```python
from build123d import *

# Parameters (mm, degrees)
CYLINDER009_R            = 2.2
CYLINDER009_DEPTH        = 20
ARRAY006_Z_COUNT         = 3
ARRAY006_Z_PITCH         = 10
CYLINDER008_R            = 1.8
CYLINDER008_DEPTH        = 10
ARRAY005_X_COUNT         = 2
ARRAY005_X_PITCH         = 20
ARRAY005_Y_COUNT         = 2
ARRAY005_Y_PITCH         = 20
ARRAY005_PLACEMENT_ANGLE = 90
PAD002_DEPTH             = 16


with BuildPart() as holder_insert_hole_array:
    # Cylinder009 → Cylinder009 (new body)
    with BuildSketch(Plane.XZ):
        Circle(CYLINDER009_R)
    extrude(amount=CYLINDER009_DEPTH)

    # Array006 Z: holder insert hole array ×3


with BuildPart() as holder_insert_hole_array_1:
    add(holder_insert_hole_array.part)
    with Locations(*[(0, 0, i * ARRAY006_Z_PITCH) for i in range(1, ARRAY006_Z_COUNT)]):
        add(holder_insert_hole_array.part)


with BuildPart() as holder_insert_hole_array_2:
    # Array006 placement: moved
    add(holder_insert_hole_array_1.part.moved(Location((35, 103, 71.5))))


with BuildPart() as holder_hole_fusion:
    # Cylinder008 → Cylinder008 (new body)
    with BuildSketch(Plane.XY):
        Circle(CYLINDER008_R)
    extrude(amount=CYLINDER008_DEPTH)

    # Array005 X: holder hole fusion ×2


with BuildPart() as holder_hole_fusion_1:
    add(holder_hole_fusion.part)
    with Locations(*[(i * ARRAY005_X_PITCH, 0, 0) for i in range(1, ARRAY005_X_COUNT)]):
        add(holder_hole_fusion.part)

    # Array005 Y: holder hole fusion ×2


with BuildPart() as holder_hole_fusion_2:
    add(holder_hole_fusion_1.part)
    with Locations(*[(0, i * ARRAY005_Y_PITCH, 0) for i in range(1, ARRAY005_Y_COUNT)]):
        add(holder_hole_fusion_1.part)


with BuildPart() as holder_hole_fusion_3:
    # Array005 placement: moved
    add(holder_hole_fusion_2.part.moved(Location((24, 88, 16))).rotate(Axis((24, 88, 16), (1, 0, 0)), ARRAY005_PLACEMENT_ANGLE))

    # Fusion008: union holder insert hole array
    add(holder_insert_hole_array_2.part)


with BuildPart() as holder_cut:
    # Sketch002 → Pad002 (new body, symmetric)
    with BuildSketch(Plane.YZ):
        with BuildLine():
            Line((65.267053, 48), (83, 48))
            Line((83, 48), (83, 9.6))
            Line((83, 9.6), (87, 9.6))
            Line((87, 9.6), (87, 40.719632))
            ThreePointArc((94.280368, 48), (89.13237, 45.86763), (87, 40.719632))
            Line((94.280368, 48), (95.267053, 48))
            Line((95.267053, 48), (95.267053, 98))
            ThreePointArc((95.267053, 98), (92.767053, 100.5), (90.267053, 98))
            Line((90.267053, 98), (90.267053, 53))
            Line((90.267053, 53), (70.267053, 53))
            Line((70.267053, 53), (70.267053, 79))
            ThreePointArc((70.267053, 79), (67.767053, 81.5), (65.267053, 79))
            Line((65.267053, 79), (65.267053, 48))
        make_face()
    extrude(amount=PAD002_DEPTH, both=True)


with BuildPart() as holder_cut_1:
    # Body002 placement: moved
    add(holder_cut.part.moved(Location((35, 0, 0))))

    # Cut001006: cut holder hole fusion
    add(holder_hole_fusion_3.part, mode=Mode.SUBTRACT)


solid = holder_cut_1.part
```
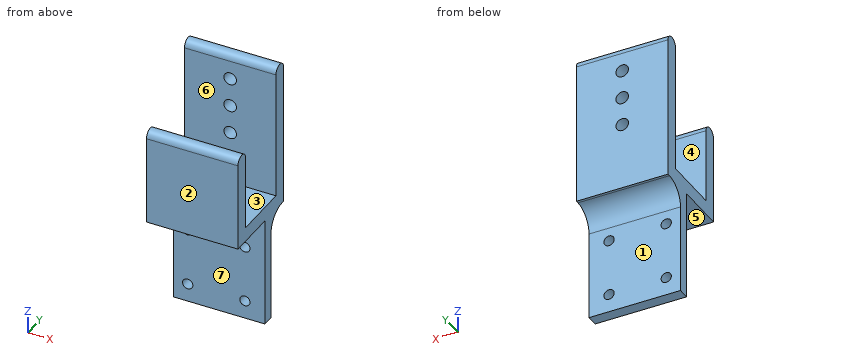
Check sheet for the modelled part. Datum: model origin and axes. Units: mm. Face numbers are marked on the shaded views. A direction names the side the tool comes from. Round coordinates to 2 decimals unless told otherwise and drop trailing zeros. Loops run counter-clockwise (first coordinate to the right, second up) from the corner with the lowest first, then second, coordinate; pieces in that order, holes last. Notation, with made-up numbers: (59, 32) -> (107, 32) arc R9 ccw to (107, 45) -> close; hole circle Ø1 at (52.5, 68.25). An arc over 180 degrees is marked (long way). Answer in a Markdown table with one row per item.
Q1. Sectioned sample at C-C on x = 35. Enter the section's corners in (y, z).
Data:
| item | result |
|---|---|
| outline | (65.27, 48) -> (83, 48) -> (83, 9.6) -> (87, 9.6) -> (87, 40.72) arc R7.28 cw to (94.28, 48) -> (95.27, 48) -> (95.27, 69.3) -> (90.27, 69.3) -> (90.27, 53) -> (70.27, 53) -> (70.27, 79) arc R2.5 ccw to (65.27, 79) -> close; (90.27, 73.7) -> (95.27, 73.7) -> (95.27, 79.3) -> (90.27, 79.3) -> close; (90.27, 83.7) -> (95.27, 83.7) -> (95.27, 89.3) -> (90.27, 89.3) -> close; (90.27, 93.7) -> (95.27, 93.7) -> (95.27, 98) arc R2.5 ccw to (90.27, 98) -> close |
Q2. Go/stop test with flat-tipped pins: P1, Ø1, axis at x = 43.5, y = 74, coming from the +Z side; P2, Ø12, axis at y = 89, z = 37, coming from the +X side; P3, Ø4, axis at x = 24, z = 16, coming from the -Y side; P4, Ø3, axis at x = 44, z = 36, coming from the +Y side. Record where each tip stops, or that it passes through.
Data:
| item | result |
|---|---|
| P1 | stops at z = 53 |
| P2 | stops at x = 51 |
| P3 | stops at y = 83 |
| P4 | passes through |
Q3. Set-up check for the marked faces 1, 2 and 3: record each of +Z, -Z, +X, -X, +Y, -Y from which the full face is reachable in a straight line by a thin tool's end or side.
Data:
| item | result |
|---|---|
| face 1 | -Z, +X, -X, +Y |
| face 2 | +Z, -Z, +X, -X, -Y |
| face 3 | +Z, +X, -X |
Q4. Release check for a two-part mould opening along Y. For the marked faces 4, 5, 6 and 7 record: released by +Y, released by -Y, zero draft, split by the parting line, or undercut.
Data:
| item | result |
|---|---|
| face 4 | undercut |
| face 5 | zero draft |
| face 6 | undercut |
| face 7 | released by -Y |
Q5. Sectioned sample at B-B on x = 44. Enter the section's corners in (y, z).
Data:
| item | result |
|---|---|
| outline | (65.27, 48) -> (83, 48) -> (83, 37.8) -> (87, 37.8) -> (87, 40.72) arc R7.28 cw to (94.28, 48) -> (95.27, 48) -> (95.27, 98) arc R2.5 ccw to (90.27, 98) -> (90.27, 53) -> (70.27, 53) -> (70.27, 79) arc R2.5 ccw to (65.27, 79) -> close; (83, 9.6) -> (87, 9.6) -> (87, 14.2) -> (83, 14.2) -> close; (83, 17.8) -> (87, 17.8) -> (87, 34.2) -> (83, 34.2) -> close |
Q6. Thickness scan on L1, parallel to X at y = 84.3, z = 36; L2, parallel to Z at x = 24, y = 84.7; L3, parallel to Y at x = 40, z = 62. Record the ranges inside material, lowest first.
Data:
| item | result |
|---|---|
| L1 | x = 19 to 22.2, 25.8 to 42.2, 45.8 to 51 |
| L2 | z = 9.6 to 14.2, 17.8 to 34.2, 37.8 to 53 |
| L3 | y = 65.27 to 70.27, 90.27 to 95.27 |
Q7. Sectioned sample at A-A on z = 71.5. Enter the section's corners in (x, y), then the cut area to 3 significant figures.
Data:
| item | result |
|---|---|
| outline | (19, 65.27) -> (51, 65.27) -> (51, 70.27) -> (19, 70.27) -> close; (19, 90.27) -> (32.8, 90.27) -> (32.8, 95.27) -> (19, 95.27) -> close; (37.2, 90.27) -> (51, 90.27) -> (51, 95.27) -> (37.2, 95.27) -> close |
| area | 298 mm^2 |
Q8. Sectioned sample at D-D on z = 91.5. Enter the section's corners in (x, y), then the cut area to 3 significant figures.
Data:
| item | result |
|---|---|
| outline | (19, 90.27) -> (32.8, 90.27) -> (32.8, 95.27) -> (19, 95.27) -> close; (37.2, 90.27) -> (51, 90.27) -> (51, 95.27) -> (37.2, 95.27) -> close |
| area | 138 mm^2 |
